Can you work these out from the model? Positions are in its coordinate system, mm. Face numbers are marked on the shaded views. A direction names the side the tool comes from. Coordinates: 2 decimals unless noted, no trailing zeros. Write each loop counter-clockwise with the first axis right and the second up, starting at its lowest first coordinate (ties: lowest second). Pieces come first, ordered by that corner, then holes. Notation, with made-up numbers: M -18,-25.5 L 9,-25.5 A18 ccw 9,6.5 Z; hole C -14,-3.5 d1. An arc over 180 degrees is marked long. Use one line per item in the form item = value. Start each with the question number.
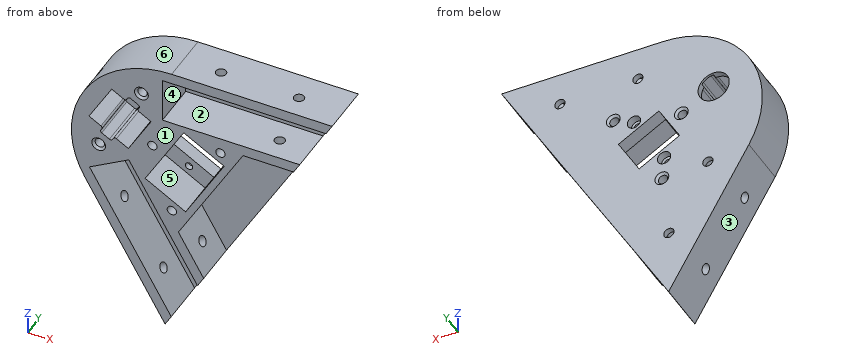
```python
from build123d import *

# Parameters (mm, degrees)
BOSS_EXTRUDE1_DEPTH      = 23
SKETCH2_W                = 100.4
SKETCH2_H                = 20.4
CUT_EXTRUDE2_DEPTH       = 20.4
CUT_EXTRUDE3_DEPTH       = 20
SKETCH7_R                = 2.3
CUT_EXTRUDE6_DEPTH       = 10
SKETCH8_R                = 2.3
CUT_EXTRUDE7_DEPTH       = 10
FILLET3_R                = 45
CUT_EXTRUDE11_DEPTH      = 200.759855827
CUT_EXTRUDE11_DEPTH_BACK = 200.759855827
CUT_EXTRUDE10_DEPTH      = 20
SKETCH32_R               = 2.3
CUT_EXTRUDE18_DEPTH      = 10
SKETCH33_R               = 2.3
CUT_EXTRUDE19_DEPTH      = 10
SKETCH34_R               = 2.3
CUT_EXTRUDE20_DEPTH      = 149.465956609
SKETCH35_R               = 4
CUT_EXTRUDE21_DEPTH      = 152.333845776
SKETCH36_R               = 2.1
CUT_EXTRUDE22_DEPTH      = 200.759855838
SKETCH38_R               = 2.3
CUT_EXTRUDE24_DEPTH      = 10
BOSS_EXTRUDE2_DEPTH      = 6
SKETCH40_R               = 1.65
CUT_EXTRUDE25_DEPTH      = 200.158228561
SKETCH41_R               = 3
CUT_EXTRUDE26_DEPTH      = 3.5
SKETCH42_R               = 2.1
CUT_EXTRUDE27_DEPTH      = 200.759855838
CHAMFER2_SIZE            = 1
SKETCH43_R               = 2.1
CUT_EXTRUDE28_DEPTH      = 15
CHAMFER3_SIZE            = 1
SKETCH45_R               = 2.3
CUT_EXTRUDE29_DEPTH      = 130.123625221
SKETCH46_R               = 4
CUT_EXTRUDE30_DEPTH      = 127.307236488
SKETCH47_R               = 7
CUT_EXTRUDE31_DEPTH      = 10
CUT_EXTRUDE32_DEPTH      = 20
CUT_EXTRUDE32_DEPTH_BACK = 2
FILLET4_R                = 1


with BuildPart() as part:
    # Sketch1 → Boss-Extrude1 (new body)
    with BuildSketch(Plane(origin=(0, 0, 0), x_dir=(1, 0, 0), z_dir=(0, 1, 0))):
        Polygon((0, 0), (150, 0), (75, 129.903810568), align=None)
    extrude(amount=BOSS_EXTRUDE1_DEPTH)

    # Sketch2 → Cut-Extrude2 (cut)
    with BuildSketch(Plane(origin=(0, 0, 0), x_dir=(1, 0, 0), z_dir=(0, 1, 0))):
        Polygon((108.923840175, 138.261625339), (58.723840175, 51.312674799), (41.056921938, 61.512674799), (91.256921938, 148.461625339), align=None)
        with Locations((124, 15)):
            Rectangle(SKETCH2_W, SKETCH2_H)
    extrude(amount=CUT_EXTRUDE2_DEPTH, mode=Mode.SUBTRACT)

    # Sketch4 → Cut-Extrude3 (cut)
    with BuildSketch(Plane(origin=(0, 0, 0), x_dir=(1, 0, 0), z_dir=(0, 1, 0))):
        Polygon((58.515583945, 45.561933634), (40.848665708, 35.361933634), (51.048665708, 17.695015397), (68.715583945, 27.895015397), align=None)
    extrude(amount=CUT_EXTRUDE3_DEPTH, mode=Mode.SUBTRACT)

    # Sketch7 → Cut-Extrude6 (cut)
    with BuildSketch(Plane(origin=(0, 0, 0), x_dir=(-0.4999999999999978, 0, 0.86602540378444), z_dir=(-0.86602540378444, 0, -0.4999999999999978))):
        with Locations((-130, 10)):
            Circle(SKETCH7_R)
        with Locations((-95, 10)):
            Circle(SKETCH7_R)
    extrude(amount=-CUT_EXTRUDE6_DEPTH, mode=Mode.SUBTRACT)

    # Sketch8 → Cut-Extrude7 (cut)
    with BuildSketch(Plane.XY):
        with Locations((130, 10)):
            Circle(SKETCH8_R)
        with Locations((95, 10)):
            Circle(SKETCH8_R)
    extrude(amount=-CUT_EXTRUDE7_DEPTH, mode=Mode.SUBTRACT)

    # Fillet3
    fillet3_edges = [part.edges().sort_by_distance(p)[0] for p in [
        (0, 11.5, 0),
    ]]
    fillet(fillet3_edges, radius=FILLET3_R)

    # Sketch22 → Cut-Extrude11 (cut, two sides: drawn at the far end of the back side and taken through both)
    with BuildSketch(Plane.XZ.offset(-CUT_EXTRUDE11_DEPTH_BACK)):
        Polygon((83.35335133, -28.147760515), (66.05335133, -58.112239485), (84.23988481, -68.612239485), (101.53988481, -38.647760515), align=None)
    extrude(amount=CUT_EXTRUDE11_DEPTH + CUT_EXTRUDE11_DEPTH_BACK, mode=Mode.SUBTRACT)

    # Sketch21 → Cut-Extrude10 (cut)
    with BuildSketch(Plane.XZ):
        Polygon((132.679491924, -30), (109.996773286, -30), (80.979148757, -80.26), (92.320508076, -99.903810568), align=None)
    extrude(amount=-CUT_EXTRUDE10_DEPTH, mode=Mode.SUBTRACT)

    # Sketch32 → Cut-Extrude18 (cut)
    with BuildSketch(Plane(origin=(0, 0, -30), x_dir=(-1, 0, 0), z_dir=(0, 0, -1))):
        with Locations((-121.338132605, 10)):
            Circle(SKETCH32_R)
    extrude(amount=-CUT_EXTRUDE18_DEPTH, mode=Mode.SUBTRACT)

    # Sketch33 → Cut-Extrude19 (cut)
    with BuildSketch(Plane(origin=(25.980762114, 0, 15), x_dir=(0.4999999999999997, 0, -0.8660254037844388), z_dir=(0.8660254037844389, 0, 0.49999999999999983))):
        with Locations((121.338132605, 10)):
            Circle(SKETCH33_R)
    extrude(amount=-CUT_EXTRUDE19_DEPTH, mode=Mode.SUBTRACT)

    # Sketch34 → Cut-Extrude20 (cut, through all)
    with BuildSketch(Plane(origin=(45.948665708, 0, -26.528474516), x_dir=(-0.5000000000000001, 0, -0.8660254037844386), z_dir=(0.8660254037844386, 0, -0.5000000000000001))):
        with Locations((0, 10)):
            Circle(SKETCH34_R)
    extrude(amount=-CUT_EXTRUDE20_DEPTH, mode=Mode.SUBTRACT)

    # Sketch35 → Cut-Extrude21 (cut, through all)
    with BuildSketch(Plane(origin=(43.350589497, 0, -25.028474516), x_dir=(-0.5000000000000001, 0, -0.8660254037844386), z_dir=(0.8660254037844386, 0, -0.5000000000000001))):
        with Locations((0, 10)):
            Circle(SKETCH35_R)
    extrude(amount=-CUT_EXTRUDE21_DEPTH, mode=Mode.SUBTRACT)

    # Sketch36 → Cut-Extrude22 (cut, through all)
    with BuildSketch(Plane(origin=(0, 23, 0), x_dir=(1, 0, 0), z_dir=(0, 1, 0))):
        with Locations(Location((69.282032303, 40, 0), (0, 0, 270))):
            Circle(SKETCH36_R)
    extrude(amount=-CUT_EXTRUDE22_DEPTH, mode=Mode.SUBTRACT)

    # Sketch38 → Cut-Extrude24 (cut)
    with BuildSketch(Plane.XZ.offset(-20.4)):
        with Locations(Location((88.8, -15, 0), (0, 0, 270))):
            Circle(SKETCH38_R)
        with Locations(Location((123.8, -15, 0), (0, 0, 270))):
            Circle(SKETCH38_R)
        with Locations(Location((57.390381057, -69.403055856, 0), (0, 0, 270))):
            Circle(SKETCH38_R)
        with Locations(Location((74.890381057, -99.713944989, 0), (0, 0, 270))):
            Circle(SKETCH38_R)
    extrude(amount=-CUT_EXTRUDE24_DEPTH, mode=Mode.SUBTRACT)

    # Sketch39 → Boss-Extrude2 (add)
    with BuildSketch(Plane(origin=(0, 23, 0), x_dir=(1, 0, 0), z_dir=(0, 1, 0))):
        Polygon((66.05335133, 58.112239485), (84.23988481, 68.612239485), (88.23988481, 61.684036255), (70.05335133, 51.184036255), align=None)
        Polygon((101.53988481, 38.647760515), (83.35335133, 28.147760515), (79.35335133, 35.075963745), (97.53988481, 45.575963745), align=None)
    extrude(amount=-BOSS_EXTRUDE2_DEPTH)

    # Sketch40 → Cut-Extrude25 (cut, through all)
    with BuildSketch(Plane.XZ.offset(-17)):
        with Locations(Location((90.54661807, -36.688657049, 0), (0, 0, 270))):
            Circle(SKETCH40_R)
        with Locations(Location((77.04661807, -60.071342951, 0), (0, 0, 270))):
            Circle(SKETCH40_R)
    extrude(amount=-CUT_EXTRUDE25_DEPTH, mode=Mode.SUBTRACT)

    # Sketch41 → Cut-Extrude26 (cut)
    with BuildSketch(Plane(origin=(0, 23, 0), x_dir=(1, 0, 0), z_dir=(0, 1, 0))):
        with Locations(Location((77.04661807, 60.071342951, 0), (0, 0, 270))):
            Circle(SKETCH41_R)
        with Locations(Location((90.54661807, 36.688657049, 0), (0, 0, 270))):
            Circle(SKETCH41_R)
    extrude(amount=-CUT_EXTRUDE26_DEPTH, mode=Mode.SUBTRACT)

    # Sketch42 → Cut-Extrude27 (cut, through all)
    with BuildSketch(Plane(origin=(0, 23, 0), x_dir=(1, 0, 0), z_dir=(0, 1, 0))):
        with Locations(Location((99.860934211, 32.446784409, 0), (0, 0, 270))):
            Circle(SKETCH42_R)
        with Locations(Location((78.030206675, 70.258713668, 0), (0, 0, 270))):
            Circle(SKETCH42_R)
    extrude(amount=-CUT_EXTRUDE27_DEPTH, mode=Mode.SUBTRACT)

    # Chamfer2
    chamfer2_edges = [part.edges().sort_by_distance(p)[0] for p in [
        (69.282032303, 23, -42.1),
        (99.860934211, 23, -34.546784409),
        (78.030206675, 23, -72.358713668),
    ]]
    chamfer(chamfer2_edges, length=CHAMFER2_SIZE)

    # Sketch43 → Cut-Extrude28 (cut)
    with BuildSketch(Plane.XZ):
        with Locations(Location((64.382124827, -15.000786763, 0), (0, 0, 270))):
            Circle(SKETCH43_R)
        with Locations(Location((45.182124827, -48.256162268, 0), (0, 0, 270))):
            Circle(SKETCH43_R)
    extrude(amount=-CUT_EXTRUDE28_DEPTH, mode=Mode.SUBTRACT)

    # Chamfer3
    chamfer3_edges = [part.edges().sort_by_distance(p)[0] for p in [
        (64.382124827, 0, -12.900786763),
        (45.182124827, 0, -46.156162268),
    ]]
    chamfer(chamfer3_edges, length=CHAMFER3_SIZE)

    # Sketch45 → Cut-Extrude29 (cut, through all)
    with BuildSketch(Plane(origin=(63.615583945, 0, -36.728474516), x_dir=(0.5, 0, 0.8660254037844386), z_dir=(-0.8660254037844387, 0, 0.5000000000000001))):
        with Locations(Location((0, 10, 0), (0, 0, 180))):
            Circle(SKETCH45_R)
    extrude(amount=-CUT_EXTRUDE29_DEPTH, mode=Mode.SUBTRACT)

    # Sketch46 → Cut-Extrude30 (cut, through all)
    with BuildSketch(Plane(origin=(66.213660157, 0, -38.228474516), x_dir=(0.5, 0, 0.8660254037844386), z_dir=(-0.8660254037844387, 0, 0.5000000000000001))):
        with Locations(Location((0, 10, 0), (0, 0, 180))):
            Circle(SKETCH46_R)
    extrude(amount=-CUT_EXTRUDE30_DEPTH, mode=Mode.SUBTRACT)

    # Sketch47 → Cut-Extrude31 (cut)
    with BuildSketch(Plane.XZ.offset(-20)):
        with Locations(Location((54.782124827, -31.628474516, 0), (0, 0, 270))):
            Circle(SKETCH47_R)
    extrude(amount=-CUT_EXTRUDE31_DEPTH, mode=Mode.SUBTRACT)

    # Sketch48 → Cut-Extrude32 (cut, two sides: drawn at the far end of the back side and taken through both)
    with BuildSketch(Plane.XZ.offset(-20).offset(-CUT_EXTRUDE32_DEPTH_BACK)):
        Polygon((58.684048615, -18.870144266), (45.684048615, -41.386804765), (50.880201038, -44.386804765), (63.880201038, -21.870144266), align=None)
    extrude(amount=CUT_EXTRUDE32_DEPTH + CUT_EXTRUDE32_DEPTH_BACK, mode=Mode.SUBTRACT)

    # Fillet4
    fillet4_edges = [part.edges().sort_by_distance(p)[0] for p in [
        (62.480201038, 10, -24.295015397),
        (52.280201038, 10, -41.961933634),
        (63.880201038, 11, -21.870144266),
        (47.084048615, 10, -38.961933634),
        (57.284048615, 10, -21.295015397),
        (45.684048615, 11, -41.386804765),
        (58.684048615, 11, -18.870144266),
        (50.880201038, 11, -44.386804765),
    ]]
    fillet(fillet4_edges, radius=FILLET4_R)


solid = part.part
```
1) If we mould it in two halves opening along Z, with no side actions, what happens to the marked faces 1, 2 and 3? For each: +Z half, -Z half, draft (parallel to the pull), parting line (faces both ways), or undercut.
2) Which directions (+Z, -Z, +X, -X, +Y, -Y) give clear straight access to the entire face, cutting with the end or side of a thin tool? Please do the marked faces 4, 5 and 6.
3) Suppose I cut it at B-B on x = 130. Please give me the cut outline in (y, z).
4) Suppose I cut it at A-A on y = 10. State how many separate pieces and enclosed holes the cut face has, and give its area (3 significant figures).
5) Please list where these lines run through material, in increasing order: line 1 (Z direction, x = 113, y = 15.25); line 2 (Z direction, x = 94, y = 4.75); line 3 (X direction, y = 21.1, z = -15).
6) Will these pins go through, and if not, where does the flat tip stop? pin 1 Ø5 at (x, z) = (69.28, -40) entering from +Y; pin 2 Ø1 at (y, z) = (16, -97) entering from +X; pin 3 Ø10 at (y, z) = (9.5, -99) entering from -X; pin 4 Ø5 at (x, z) = (69.28, -40) entering from -Y.
Computed values:
q1.face_1 = draft
q1.face_2 = undercut
q1.face_3 = -Z half
q2.face_4 = +X, -Y
q2.face_5 = -Y
q2.face_6 = -X, +Y, -Y
q3.outline = M 0,-30 L 20,-30 L 20,-34.64 L 23,-34.64 L 23,0 L 12.3,0 L 12.3,-4.8 L 20.4,-4.8 L 20.4,-25.2 L 0,-25.2 Z; M 0,-4.8 L 7.7,-4.8 L 7.7,0 L 0,0 Z
q4.separate_pieces = 8
q4.enclosed_holes = 4
q4.area = 2,700 mm²
q5.line_1 = -30 to -25.2, -4.8 to 0
q5.line_2 = -57.71 to -51.71, -34.29 to -25.2, -4.8 to 0
q5.line_3 = 44.4 to 86.5, 91.1 to 121.5, 126.1 to 141.34
q6.pin_1 = 22.4
q6.pin_2 = 90.93
q6.pin_3 = 54.27
q6.pin_4 = 0
